Design review of the part built by this model. Coordinates are the model's own, in mm. A direction names the side the tool comes from. Give positions to 0.01 mm unless a question says otherwise; leave off trailing zeros. Loops run counter-clockwise (first coordinate to the right, second up) from the corner with the lowest first, then second, coordinate; pieces in that order, holes last. Notation, with made-up numbers: (-12.5, 23.25) -> (23.5, 23.25) arc R8 ccw to (23.5, 29.25) -> close; hole circle Ø9 at (-20.5, 5.5). An arc over 180 degrees is marked (long way). Use CSV: the item, a comma, the result in double quotes. Start each with the question number.
Item 1: We need section A-A (x = -852). State the section outline as (y, z) points, plus the area to 3 significant figures.
Item 2: Wall thickness on line 1 along Z through (x, y) = (-566, -863.5); line 2 along Y through (x, z) = (-551, -490); line 3 along Z through (x, y) = (-947.5, -1955.5): over which ranges is each line inside the solid? List them lowest first. Write a range as from..to.
Item 3: We need section C-C (x = -293). State the section outline as (y, z) points.
Item 4: We need section D-D (x = -1028.5). State the section outline as (y, z) points, plus the area to 3 significant figures.
Item 5: Clearance check with flat-ended pins moving along their axes: pin 1 (1 mm diameter, centred on x = -638.5, y = -510, fed in from -Z); pin 2 (8 mm diameter, centred on x = -238, z = 368, fed in from +Y). State where each tip first meets the part, or that it passes through.
Item 6: We need section B-B (z = -18). State the section outline as (x, y) points, plus the area to 3 significant figures.
Item 7: For faces 1 (the face through (-154.343, -1893, 466)), 2 (the face through (-550, -1400, -229)), 3 (the face through (-429, -2400, -149)), 4 (the face through (-554.343, -1893, 117)), list the 3-axis set-ups (+Z, -Z, +X, -X, +Y, -Y) from which the entire face can be reached by the end or side of a thin tool; tool diameter is ignored.
from build123d import *

# Parameters (mm, degrees)
F1_DEPTH = 2400
F2_W     = 1000
F2_H     = 200
F3_DEPTH = 1000
F5_DEPTH = 1000


with BuildPart() as f1:
    # F0 (on Front) → F1 (new body)
    with BuildSketch(Plane.XZ):
        Polygon((-1154.342916, 315.182347), (-154.342916, 315.182347), (-154.342916, -584.817653), (45.657084, -584.817653), (45.657084, 515.182347), (-1154.342916, 515.182347), align=None)
    extrude(amount=F1_DEPTH)

    # F2 (on face) → F3 (cut)
    with BuildSketch(Plane.XZ.offset(2400)):
        with Locations((-654.342916, 415.182347)):
            Rectangle(F2_W, F2_H)
    extrude(amount=-F3_DEPTH, mode=Mode.SUBTRACT)

    # F4 (on face) → F5 (join)
    with BuildSketch(Plane.XZ.offset(1400)):
        Polygon((-954.342916, -384.817653), (-1154.342916, -384.817653), (-1154.342916, -584.817653), (-154.342916, -584.817653), (-154.342916, 415.182347), (-354.342916, 415.182347), (-354.342916, 215.182347), (-554.342916, 215.182347), (-554.342916, 15.182347), (-754.342916, 15.182347), (-754.342916, -184.817653), (-954.342916, -184.817653), align=None)
    extrude(amount=F5_DEPTH)


solid = f1.part
Results found:
1,outline,"(-2400, -584.82) -> (-1400, -584.82) -> (-1400, -184.82) -> (-2400, -184.82) -> close; (-1400, 315.18) -> (0, 315.18) -> (0, 515.18) -> (-1400, 515.18) -> close"
1,area,"680,000 mm²"
2,line 1,"315.18..515.18"
2,line 2,"-2400..-1400"
2,line 3,"-584.82..-184.82"
3,outline,"(-2400, -584.82) -> (-1400, -584.82) -> (-1400, 315.18) -> (0, 315.18) -> (0, 515.18) -> (-1400, 515.18) -> (-1400, 415.18) -> (-2400, 415.18) -> close"
4,outline,"(-2400, -584.82) -> (-1400, -584.82) -> (-1400, -384.82) -> (-2400, -384.82) -> close; (-1400, 315.18) -> (0, 315.18) -> (0, 515.18) -> (-1400, 515.18) -> close"
4,area,"480,000 mm²"
5,pin 1,"z = 315.18"
5,pin 2,"y = 0"
6,outline,"(-754.34, -2400) -> (45.66, -2400) -> (45.66, 0) -> (-154.34, 0) -> (-154.34, -1400) -> (-754.34, -1400) -> close"
6,area,"1,080,000 mm²"
7,face 1,"+Z, -X, -Y"
7,face 2,"-Z, -X, +Y"
7,face 3,"+Z, -Z, +X, -X, -Y"
7,face 4,"+Z, -X, +Y, -Y"
